from build123d import *

# Parameters (mm, degrees)
SKETCH1_W           = 32
SKETCH1_H           = 32
SKETCH1_R           = 1.3
BOSS_EXTRUDE1_DEPTH = 1.6
SKETCH2_W           = 16.2
SKETCH2_H           = 16.2
BOSS_EXTRUDE2_DEPTH = 7.86


with BuildPart() as part:
    # Sketch1 → Boss-Extrude1 (new body)
    with BuildSketch(Plane(origin=(0, 0, 0), x_dir=(1, 0, 0), z_dir=(0, 1, 0))):
        Rectangle(SKETCH1_W, SKETCH1_H)
        with Locations((-13.7, 13.7)):
            Circle(SKETCH1_R, mode=Mode.SUBTRACT)
        with Locations((13.7, 13.7)):
            Circle(SKETCH1_R, mode=Mode.SUBTRACT)
        with Locations((13.7, -13.7)):
            Circle(SKETCH1_R, mode=Mode.SUBTRACT)
        with Locations((-13.7, -13.7)):
            Circle(SKETCH1_R, mode=Mode.SUBTRACT)
    extrude(amount=BOSS_EXTRUDE1_DEPTH)

    # Sketch2 → Boss-Extrude2 (add)
    with BuildSketch(Plane(origin=(0, 1.6, 0), x_dir=(1, 0, 0), z_dir=(0, 1, 0))):
        Rectangle(SKETCH2_W, SKETCH2_H)
    extrude(amount=BOSS_EXTRUDE2_DEPTH)

    # Sketch4 → Revolve3 (revolve)
    with BuildSketch(Plane.XY):
        Polygon((0, 9.46), (0, 24.31), (8.5, 24.31), (8.5, 19.81), (6, 19.81), (6, 16.06), (8.1, 16.06), (8.1, 9.46), align=None)
        with BuildLine():
            Line((0, 25.81), (0, 24.31))
            Line((0, 24.31), (7, 24.31))
            ThreePointArc((7, 24.31), (3.579455266, 25.43079124), (0, 25.81))
        make_face()
    revolve(axis=Axis((0, 9.46, 0), (0, 1, 0)))


solid = part.part
Part model, mm, in its own coordinate system. A direction names the side the tool comes from. Coordinates: 2 decimals unless noted, no trailing zeros. Loops run counter-clockwise (first coordinate to the right, second up) from the corner with the lowest first, then second, coordinate; pieces in that order, holes last. Notation, with made-up numbers: (3.25, 22.5) -> (21.25, 22.5) arc R20 ccw to (21.25, 39.5) -> close; hole circle Ø1 at (51.25, 67.5). An arc over 180 degrees is marked (long way). Use a Markdown table: item, result. Add a question column.
Item 1: Pull direction X, two halves, no side cores. Call faces 5 (the flat face through (-2, 24.31, -7)), 6 (the cylindrical face through (-12.46, 0.79, -14.09)), 7 (the cylindrical face through (-1.756, 12.714, 7.907)): +X half, -X half, draft (parallel to the pull), parting line (faces both ways), or undercut.
Item 2: Probe probe 1 along X at (y, z) = (1.3, 13.7); probe 2 along Y at (x, z) = (1.5, 8); probe 3 along Z at (x, y) = (5, 6.25). List the from-to ranges inside material, lowest first.
Item 3: Which spindle directions (+Z, -Z, +X, -X, +Y, -Y) get a long thin tool onto all of the face, cutting with end or side? Do faces 1 (the flat face through (0, 5, 8.1)), 2 (the cylindrical face through (-6, 18, 0)), 3 (the flat face through (6, 9.46, -6)), 4 (the flat face through (-8.1, 5, 0)). Say none if no direction does.
Item 4: Band-saw the part on B-B on y = 14. Write the cut outline in (x, z).
Item 5: Band-saw the part on D-D on x = 3. Write the cut outline in (y, z), plus the area to 3 significant figures.
Item 6: Band-saw the part on A-A on x = 13.7. Write the cut outline in (y, z).
Item 7: Flat gauge pins, fed straight in: P1, Ø2.5, axis at x = 13.7, z = -13.7, coming from the +Y side; P2, Ø8.5, axis at x = -4, z = -2, coming from the +Y side; P3, Ø6, axis at x = -7, y = 7.5, coming from the -Z side; P4, Ø5, axis at x = -4, z = 0.5, coming from the +Y side. Where does each tip first touch, or does it go through?
Geometry says:
| question | item | result |
|---|---|---|
| 1 | face 5 | draft |
| 1 | face 6 | undercut |
| 1 | face 7 | parting line |
| 2 | probe 1 | -16 to -15, -12.4 to 12.4, 15 to 16 |
| 2 | probe 2 | 0 to 9.46, 19.81 to 24.31 |
| 2 | probe 3 | -8.1 to 8.1 |
| 3 | face 1 | +Z, +X, -X |
| 3 | face 2 | none |
| 3 | face 3 | -Z, +X |
| 3 | face 4 | +Z, -Z, -X |
| 4 | outline | circle Ø16.2 at (0, 0) |
| 5 | outline | (0, -16) -> (1.6, -16) -> (1.6, -8.1) -> (9.46, -8.1) -> (9.46, -7.52) -> (16.06, -7.52) -> (16.06, -5.2) -> (19.81, -5.2) -> (19.81, -7.95) -> (24.31, -7.95) -> (24.31, -6.32) arc R16.82 ccw to (24.31, 6.32) -> (24.31, 7.95) -> (19.81, 7.95) -> (19.81, 5.2) -> (16.06, 5.2) -> (16.06, 7.52) -> (9.46, 7.52) -> (9.46, 8.1) -> (1.6, 8.1) -> (1.6, 16) -> (0, 16) -> close |
| 5 | area | 399 mm² |
| 6 | outline | (0, -16) -> (1.6, -16) -> (1.6, -15) -> (0, -15) -> close; (0, -12.4) -> (1.6, -12.4) -> (1.6, 12.4) -> (0, 12.4) -> close; (0, 15) -> (1.6, 15) -> (1.6, 16) -> (0, 16) -> close |
| 7 | P1 | through |
| 7 | P2 | y = 25.81 |
| 7 | P3 | z = -8.1 |
| 7 | P4 | y = 25.74 |
